from build123d import *

# Parameters (mm, degrees)
SKETCH_2_W          = 90
SKETCH_2_H          = 36
EXTRUDE_1_DEPTH     = 32
SKETCH_3_W          = 9
SKETCH_3_H          = 24
CUT_EXTRUDE_1_DEPTH = 59.077534383
SKETCH_4_W          = 9
SKETCH_4_H          = 24
CUT_EXTRUDE_2_DEPTH = 59.077534383
SKETCH_6_R          = 11
CUT_EXTRUDE_3_DEPTH = 59.077534383
SKETCH_7_W          = 10
SKETCH_7_H          = 20
CUT_EXTRUDE_4_DEPTH = 66.916613991
SKETCH_9_W          = 12
SKETCH_9_H          = 12
CUT_EXTRUDE_5_DEPTH = 89.932558717


with BuildPart() as part:
    # Эскиз2 → Бобышка-Вытянуть1 (new body)
    with BuildSketch(Plane.XY):
        Rectangle(SKETCH_2_W, SKETCH_2_H)
    extrude(amount=EXTRUDE_1_DEPTH)

    # Эскиз3 → Вырез-Вытянуть1 (cut, through all)
    with BuildSketch(Plane.XY.offset(32)):
        with Locations((-40.5, 0)):
            Rectangle(SKETCH_3_W, SKETCH_3_H)
    extrude(amount=-CUT_EXTRUDE_1_DEPTH, mode=Mode.SUBTRACT)

    # Эскиз4 → Вырез-Вытянуть2 (cut, through all)
    with BuildSketch(Plane.XY.offset(32)):
        with Locations((40.5, 0)):
            Rectangle(SKETCH_4_W, SKETCH_4_H)
    extrude(amount=-CUT_EXTRUDE_2_DEPTH, mode=Mode.SUBTRACT)

    # Эскиз6 → Вырез-Вытянуть3 (cut, through all)
    with BuildSketch(Plane.XY.offset(32)):
        Circle(SKETCH_6_R)
    extrude(amount=-CUT_EXTRUDE_3_DEPTH, mode=Mode.SUBTRACT)

    # Эскиз7 → Вырез-Вытянуть4 (cut, through all)
    with BuildSketch(Plane(origin=(0, 18, 0), x_dir=(1, 0, 0), z_dir=(0, 1, 0))):
        with Locations((0, -16)):
            Rectangle(SKETCH_7_W, SKETCH_7_H)
    extrude(amount=-CUT_EXTRUDE_4_DEPTH, mode=Mode.SUBTRACT)

    # Эскиз9 → Вырез-Вытянуть5 (cut, through all)
    with BuildSketch(Plane.ZY.offset(36)):
        with Locations((16, 0)):
            Rectangle(SKETCH_9_W, SKETCH_9_H)
    extrude(amount=-CUT_EXTRUDE_5_DEPTH, mode=Mode.SUBTRACT)


solid = part.part
Geometry: final body of the model. Coordinates: model frame, mm. A direction names the side the tool comes from. Give positions to 0.01 mm unless a question says otherwise; leave off trailing zeros. Write each loop counter-clockwise with the first axis right and the second up, starting at its lowest first coordinate (ties: lowest second). Pieces come first, ordered by that corner, then holes. Notation, with made-up numbers: M 39.5,-9 L 78.5,-9 A32 ccw 78.5,30 Z; hole C 3,80.5 d2. An arc over 180 degrees is marked long. Answer in a Markdown table with one row per item. Add a question column.
(1) First-contact query: pin 1 (8 mm diameter, centred on y = -3, z = 12.5, fed in from -X); pin 2 (1.5 mm diameter, centred on y = -3.5, z = 27.5, fed in from +X); pin 3 (13 mm diameter, centred on x = 0, y = 0, fed in from -Z). Flat tips, straight axial feed; report the tip coordinate or a pass-through.
(2) Section B-B on z = 8.5. Return loops of the section in (x, y), and give its area (3 significant figures).
(3) Ray query, line 1 (Y direction, x = -20.5, z = 11.5); line 2 (Y direction, x = 41.5, z = 14.5); line 3 (X direction, y = -14, z = 23). Return the intervals inside material, ascending.
(4) Section D-D on y = 13. Return loops of the section in (x, z).
(5) Reachability of faces 1 (the flat face through (0, 14, 6)), 2 (the flat face through (22, -6, 16)), 3 (the flat face through (-36, 0, 9)) from +Z, -Z, +X, -X, +Y, -Y: full face, straight path, thin tool, end or side. Return the list, or none.
(6) Section A-A on y = 0. Return loops of the section in (x, z).
(7) Mould query, pull axis Y, two halves, no side actions, for faces 4 (the flat face through (-45, 15, 16)), 5 (the flat face through (22, 6, 16)), 6 (the flat face through (36, 0, 9)), 7 (the flat face through (9, 18, 16)). Classes: +Y half, -Y half, draft (parallel to the pull), parting line (faces both ways), or undercut.
(8) Section C-C on x = 0. Return loops of the section in (y, z), and give its area (3 significant figures).
Result set:
| question | item | result |
|---|---|---|
| 1 | pin 1 | stops at x = -36 |
| 1 | pin 2 | stops at x = 36 |
| 1 | pin 3 | passes through |
| 2 | outline | M -45,-18 L -5,-18 L -5,-9.8 A11 cw -5,9.8 L -5,18 L -45,18 L -45,12 L -36,12 L -36,-12 L -45,-12 Z; M 5,-18 L 45,-18 L 45,-12 L 36,-12 L 36,12 L 45,12 L 45,18 L 5,18 L 5,9.8 A11 cw 5,-9.8 Z |
| 2 | area | 2,280 mm^2 |
| 3 | line 1 | y = -18 to -6, 6 to 18 |
| 3 | line 2 | y = -18 to -12, 12 to 18 |
| 3 | line 3 | x = -45 to -5, 5 to 45 |
| 4 | outline | M -45,0 L 45,0 L 45,32 L -45,32 Z; hole M -5,6 L 5,6 L 5,26 L -5,26 Z |
| 5 | face 1 | +Y, -Y |
| 5 | face 2 | +X, -X |
| 5 | face 3 | +Z, -Z, -X |
| 6 | outline | M -36,0 L -11,0 L -11,10 L -36,10 Z; M -36,22 L -11,22 L -11,32 L -36,32 Z; M 11,0 L 36,0 L 36,10 L 11,10 Z; M 11,22 L 36,22 L 36,32 L 11,32 Z |
| 7 | face 4 | draft |
| 7 | face 5 | undercut |
| 7 | face 6 | undercut |
| 7 | face 7 | +Y half |
| 8 | outline | M -18,0 L -11,0 L -11,6 L -18,6 Z; M -18,26 L -11,26 L -11,32 L -18,32 Z; M 11,0 L 18,0 L 18,6 L 11,6 Z; M 11,26 L 18,26 L 18,32 L 11,32 Z |
| 8 | area | 168 mm^2 |
